Here's how the part is built. I have some questions about the finished solid (model axes, mm). Face numbers are marked on the shaded views. A direction names the side the tool comes from. Round coordinates to 2 decimals unless told otherwise and drop trailing zeros. Order: outer loops, then holes, each group sorted by start corner. A loop starts at its lowest first (then second) coordinate and runs counter-clockwise, first axis right, second up.
```python
from build123d import *

# Parameters (mm, degrees)
CYLINDER017_R     = 2.65
CYLINDER017_DEPTH = 2
CYLINDER016_R     = 6.55
CYLINDER016_DEPTH = 5


with BuildPart() as cylinder017:
    # Cylinder017 → Cylinder017 (new body)
    with BuildSketch(Plane.XY.offset(3)):
        Circle(CYLINDER017_R)
    extrude(amount=CYLINDER017_DEPTH)


with BuildPart() as cut028006004005015:
    # Cylinder016 → Cylinder016 (new body)
    with BuildSketch(Plane.XY):
        Circle(CYLINDER016_R)
    extrude(amount=CYLINDER016_DEPTH)

    # Cut028006004005015: cut Cylinder017
    add(cylinder017.part, mode=Mode.SUBTRACT)


with BuildPart() as cut028006004005015_1:
    # Cut028006004005015 placement: moved
    add(cut028006004005015.part.moved(Location((22, 0, 33))))


solid = cut028006004005015_1.part
```
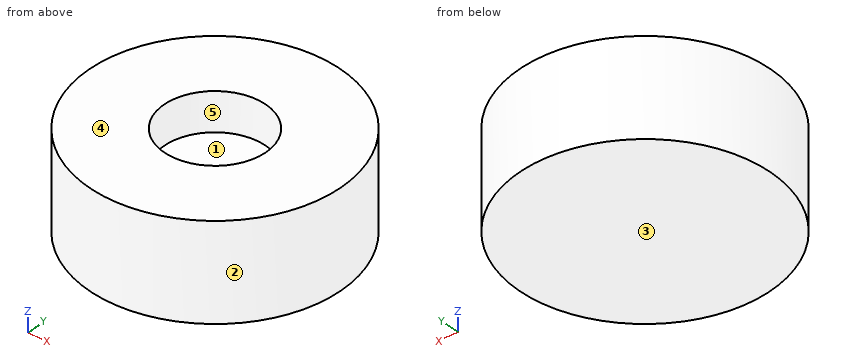
1) We'd pull the mould along Y, two halves only. Please class the marked faces 1, 2 and 3: +Y half, -Y half, draft (parallel to the pull), parting line (faces both ways), or undercut.
2) I need wall thicknesses on line 1 (Y direction, x = 22, z = 37.1); line 2 (Z direction, x = 21.5, y = -2.25); line 3 (Y direction, x = 27.5, z = 34.2). Which ranges of each line are inside material? Lowest first, please.
3) If we section it at A-A (x = 22): Write out the boundary of the cut face in (y, z), plus the area to 3 significant figures.
4) For the marked faces 4 and 5, which set-ups out of +Z, -Z, +X, -X, +Y, -Y let a thin tool reach every point of the face, with its end or its side?
5) If we section it at C-C (z = 36.25): Write out the boundary of the cut face in (x, y), plus the area to 3 significant figures.
6) If we section it at D-D (z = 33.3): Write out the boundary of the cut face in (x, y).
7) If we section it at B-B (y = 0): Write out the boundary of the cut face in (x, z).
8) I'm going to push flat-ended pins straight in: pin 1 (2 mm diameter, centred on y = 4.5, z = 35.5, fed in from +X); pin 2 (2 mm diameter, centred on x = 19, z = 36, fed in from -Y). Where does each tip first touch, or does it pass through?
Solutions:
1. face 1: undercut
1. face 2: parting line
1. face 3: draft
2. line 1: y = -6.55 to -2.65, 2.65 to 6.55
2. line 2: z = 33 to 36
2. line 3: y = -3.56 to 3.56
3. outline: (-6.55, 33) - (6.55, 33) - (6.55, 38) - (2.65, 38) - (2.65, 36) - (-2.65, 36) - (-2.65, 38) - (-6.55, 38) - close
3. area: 54.9 mm2
4. face 4: +Z, +X, -X, +Y, -Y
4. face 5: +Z
5. outline: circle Ø13.1 at (22, 0); hole circle Ø5.3 at (22, 0)
5. area: 113 mm2
6. outline: circle Ø13.1 at (22, 0)
7. outline: (15.45, 33) - (28.55, 33) - (28.55, 38) - (24.65, 38) - (24.65, 36) - (19.35, 36) - (19.35, 38) - (15.45, 38) - close
8. pin 1: stops at x = 27.54
8. pin 2: stops at y = -6.24
